Check sheet for the drawn part. Datum: minimum x, y, z corner. Units: mm. A direction names the side the tool comes from. Round coordinates to 2 decimals unless told otherwise and drop trailing zeros. Order: outer loops, then holes, each group sorted by start corner. A loop starts at its lowest first (then second) coordinate and runs counter-clockwise, first axis right, second up. Notation, with made-up numbers: (47.5, 28) - (86.5, 28) arc R36 cw to (86.5, 62) - close; hole circle Ø8 at (-19, 55). An arc over 180 degrees is marked (long way). Write each question's results on one line, items separated by ' | '.
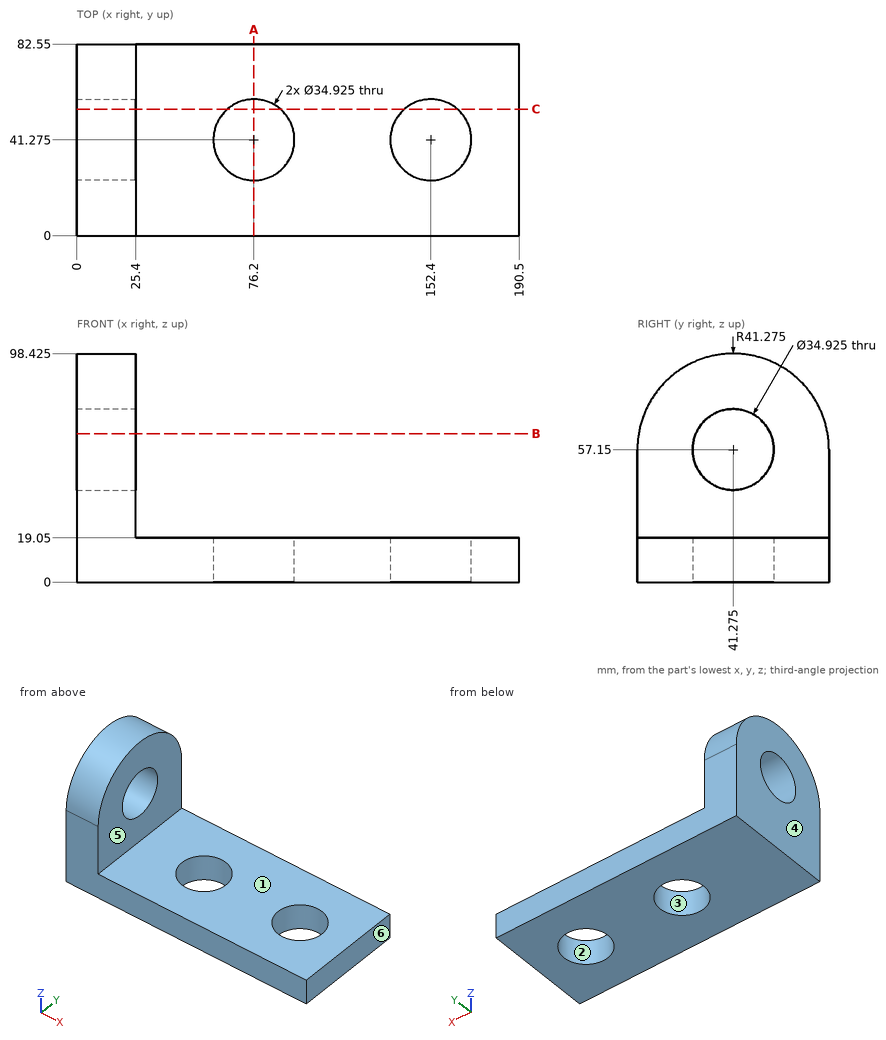
(1) Draft check along X on the marked faces 1, 2, 3 and 4. Enter one of: released by +X, released by -X, zero draft, split by the parting line, or undercut.
Answers follow:
face 1: zero draft | face 2: undercut | face 3: undercut | face 4: released by -X
(2) Depth check by flat-ended pin: pin 1 Ø4 at (x, z) = (88.5, 21.5) entering from +Y; pin 2 Ø6 at (x, y) = (134, 30) entering from +Z; pin 3 Ø3 at (y, z) = (30, 11.5) entering from -X. Enter the tip coordinate at first touch or a pass-through.
Answers follow:
pin 1: through | pin 2: z = 19.05 | pin 3: x = 0
(3) Material ranges on line 1 (Y direction, x = 76, z = 14); line 2 (X direction, y = 45, z = 12); line 3 (X direction, y = 32, z = 17.5), recorded low to high.
Answers follow:
line 1: 0 to 23.81, 58.74 to 82.55 | line 2: 0 to 59.14, 93.26 to 135.34, 169.46 to 190.5 | line 3: 0 to 61.4, 91 to 137.6, 167.2 to 190.5
(4) Section check A-A (x = 76.2). Record the cut outline in (y, z).
Answers follow:
outline: (0, 0) - (23.81, 0) - (23.81, 19.05) - (0, 19.05) - close; (58.74, 0) - (82.55, 0) - (82.55, 19.05) - (58.74, 19.05) - close
(5) Access from +Z, -Z, +X, -X, +Y, -Y to the whole of each face (thin tool, end or side, straight path). Record for the marked faces 5 and 6.
Answers follow:
face 5: +Z, +X, +Y, -Y | face 6: +Z, -Z, +X, +Y, -Y
(6) Section check C-C (y = 54.5). Record the cut outline in (x, z).
Answers follow:
outline: (0, 0) - (64.8, 0) - (64.8, 19.05) - (25.4, 19.05) - (25.4, 45.75) - (0, 45.75) - close; (0, 68.55) - (25.4, 68.55) - (25.4, 96.25) - (0, 96.25) - close; (87.6, 0) - (141, 0) - (141, 19.05) - (87.6, 19.05) - close; (163.8, 0) - (190.5, 0) - (190.5, 19.05) - (163.8, 19.05) - close
(7) Section check B-B (z = 64). Record the cut outline in (x, y).
Answers follow:
outline: (0, 0.57) - (25.4, 0.57) - (25.4, 25.21) - (0, 25.21) - close; (0, 57.34) - (25.4, 57.34) - (25.4, 81.98) - (0, 81.98) - close
